Verification items for the finished model (mm, model axes). Face numbers are marked on the shaded views. Coordinates: 2 decimals unless noted, no trailing zeros. Loops run counter-clockwise (first coordinate to the right, second up) from the corner with the lowest first, then second, coordinate; pieces in that order, holes last. Notation, with made-up numbers: (37.25, 65) - (52.25, 65) arc R19 cw to (52.25, 69) - close; hole circle Ø7 at (-25, -8). An arc over 180 degrees is marked (long way). Answer as CSV lines item,"result". Start each with the question number.
1. Release check for a two-part mould opening along Y. For the marked faces 1 and 2 record: pulls with the +Y half, pulls with the -Y half, needs draft (parallel to the pull), parting line crosses it, or undercut.
2. Cross-section at B-B (z = -2). Enter the section's corners in (x, y).
3. Cross-section at A-A (y = 1460). State how many separate pieces and enclosed holes the cut face has, plus the area to 3 significant figures.
4. Material ranges on line 1 (Y direction, x = -53, z = -130); line 2 (Y direction, x = 55.5, z = 9.5); line 3 (Z direction, x = 56.5, y = 1460), recorded low to high. Write a range as [from, to].
5. Cross-section at C-C (x = 10). Enter the section's corners in (y, z), plus the area to 3 significant figures.
6. Gauge pin test, flat ends, axial feed: P1, Ø5, axis at x = 56, z = 14, coming from the -Y side; P2, Ø8, axis at y = 513, z = -42.5, coming from the +X side; P3, Ø4, axis at x = -22.5, y = 675.5, coming from the -Z side; P4, Ø11, axis at x = -52.5, z = -0.5, coming from the +Y side. Record the tip position at first contact, or that the pin passes through.
7. Cross-section at D-D (y = 587.5). Enter the section's corners in (x, z).
```python
from build123d import *

# Parameters (mm, degrees)
BOSS_EXTRUDE1_DEPTH = 2060
SKETCH2_R           = 17.5
BOSS_EXTRUDE2_DEPTH = 10
SKETCH4_R           = 17.5
BOSS_EXTRUDE3_DEPTH = 10


with BuildPart() as part:
    # Sketch1 → Boss-Extrude1 (new body)
    with BuildSketch(Plane(origin=(0, 0, 0), x_dir=(1, 0, 0), z_dir=(0, 1, 0))):
        with BuildLine():
            Line((-45, -75), (45, -75))
            ThreePointArc((45, -75), (48.535533906, -73.535533906), (50, -70))
            Line((50, -70), (50, 70))
            ThreePointArc((50, 70), (48.535533906, 73.535533906), (45, 75))
            Line((45, 75), (-45, 75))
            ThreePointArc((-45, 75), (-48.535533906, 73.535533906), (-50, 70))
            Line((-50, 70), (-50, -70))
            ThreePointArc((-50, -70), (-48.535533906, -73.535533906), (-45, -75))
        make_face()
        with BuildLine():
            Line((-30, -60), (30, -60))
            ThreePointArc((30, -60), (33.535533906, -58.535533906), (35, -55))
            Line((35, -55), (35, 55))
            ThreePointArc((35, 55), (33.535533906, 58.535533906), (30, 60))
            Line((30, 60), (-30, 60))
            ThreePointArc((-30, 60), (-33.535533906, 58.535533906), (-35, 55))
            Line((-35, 55), (-35, -55))
            ThreePointArc((-35, -55), (-33.535533906, -58.535533906), (-30, -60))
        make_face(mode=Mode.SUBTRACT)
    extrude(amount=BOSS_EXTRUDE1_DEPTH)

    # Sketch2 → Boss-Extrude2 (add)
    with BuildSketch(Plane(origin=(50, 0, 0), x_dir=(0, 0, -1), z_dir=(1, 0, 0))):
        with BuildLine():
            Line((43.395359238, 1396.045447211), (139.154011501, 1415.94090249))
            ThreePointArc((139.154011501, 1415.94090249), (175, 1460), (139.154011501, 1504.05909751))
            Line((139.154011501, 1504.05909751), (43.395359238, 1523.954552789))
            ThreePointArc((43.395359238, 1523.954552789), (38.336590995, 1524.737951503), (33.224235348, 1525))
            Line((33.224235348, 1525), (-56.636474138, 1525))
            Line((-56.636474138, 1525), (-56.636474138, 1460))
            Line((-56.636474138, 1460), (-56.636474138, 1395))
            Line((-56.636474138, 1395), (33.224235348, 1395))
            ThreePointArc((33.224235348, 1395), (38.336590995, 1395.262048497), (43.395359238, 1396.045447211))
        make_face()
        with Locations((130, 1460)):
            Circle(SKETCH2_R, mode=Mode.SUBTRACT)
        with BuildLine():
            Line((-56.636474138, 200), (-56.636474138, 265))
            Line((-56.636474138, 265), (104.432577767, 265))
            ThreePointArc((104.432577767, 265), (110.295724617, 264.655045152), (116.07797063, 263.624940361))
            Line((116.07797063, 263.624940361), (219.31631429, 238.899952288))
            ThreePointArc((219.31631429, 238.899952288), (250, 200), (219.31631429, 161.100047712))
            Line((219.31631429, 161.100047712), (116.07797063, 136.375059639))
            ThreePointArc((116.07797063, 136.375059639), (110.295724617, 135.344954848), (104.432577767, 135))
            Line((104.432577767, 135), (-56.636474138, 135))
            Line((-56.636474138, 135), (-56.636474138, 200))
        make_face()
        with Locations((210, 200)):
            Circle(SKETCH2_R, mode=Mode.SUBTRACT)
    extrude(amount=BOSS_EXTRUDE2_DEPTH)

    # Sketch4 → Boss-Extrude3 (add)
    with BuildSketch(Plane.ZY.offset(50)):
        with BuildLine():
            Line((-219.31631429, 238.899952288), (-109.901430019, 263.757549946))
            ThreePointArc((-109.901430019, 263.757549946), (-104.397629265, 264.688416645), (-98.824367082, 265))
            Line((-98.824367082, 265), (56.64, 265))
            Line((56.64, 265), (56.64, 200))
            Line((56.64, 200), (56.64, 135))
            Line((56.64, 135), (-98.824367082, 135))
            ThreePointArc((-98.824367082, 135), (-104.397629265, 135.311583355), (-109.901430019, 136.242450054))
            Line((-109.901430019, 136.242450054), (-219.31631429, 161.100047712))
            ThreePointArc((-219.31631429, 161.100047712), (-250, 200), (-219.31631429, 238.899952288))
        make_face()
        with Locations((-210, 200)):
            Circle(SKETCH4_R, mode=Mode.SUBTRACT)
        with BuildLine():
            Line((56.64, 1460), (56.64, 1525))
            Line((56.64, 1525), (-33.220885504, 1525))
            ThreePointArc((-33.220885504, 1525), (-38.333067886, 1524.737969312), (-43.391668321, 1523.954623652))
            Line((-43.391668321, 1523.954623652), (-139.154011501, 1504.05909751))
            ThreePointArc((-139.154011501, 1504.05909751), (-175, 1460), (-139.154011501, 1415.94090249))
            Line((-139.154011501, 1415.94090249), (-43.391668321, 1396.045376348))
            ThreePointArc((-43.391668321, 1396.045376348), (-38.333067886, 1395.262030688), (-33.220885504, 1395))
            Line((-33.220885504, 1395), (56.64, 1395))
            Line((56.64, 1395), (56.64, 1460))
        make_face()
        with Locations((-130, 1460)):
            Circle(SKETCH4_R, mode=Mode.SUBTRACT)
    extrude(amount=BOSS_EXTRUDE3_DEPTH)


solid = part.part
```
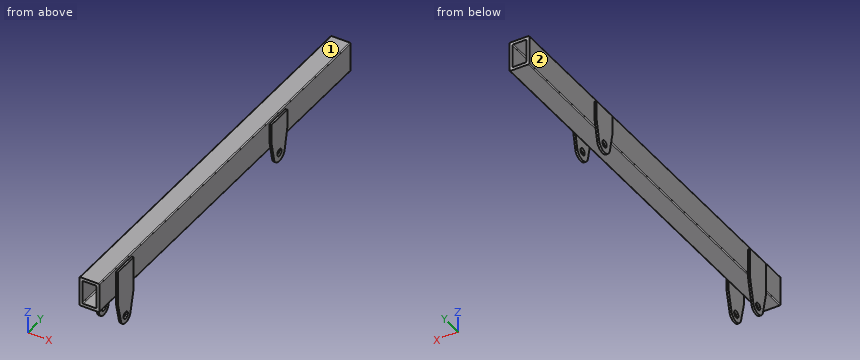
Values follow:
1,face 1,"needs draft"
1,face 2,"undercut"
2,outline,"(-60, 135) - (-50, 135) - (-50, 0) - (-35, 0) - (-35, 2060) - (-50, 2060) - (-50, 1525) - (-60, 1525) - (-60, 1395) - (-50, 1395) - (-50, 265) - (-60, 265) - close; (35, 0) - (50, 0) - (50, 135) - (60, 135) - (60, 265) - (50, 265) - (50, 1395) - (60, 1395) - (60, 1525) - (50, 1525) - (50, 2060) - (35, 2060) - close"
3,separate pieces,"3"
3,enclosed holes,"1"
3,area,"10,500 mm²"
4,line 1,"y = [140.81, 259.19], [1414.04, 1442.5], [1477.5, 1505.96]"
4,line 2,"y = [135, 265], [1395, 1525]"
4,line 3,"z = [-175, -147.5], [-112.5, 56.64]"
5,outline,"(0, -75) - (2060, -75) - (2060, -60) - (0, -60) - close; (0, 60) - (2060, 60) - (2060, 75) - (0, 75) - close"
5,area,"61,800 mm²"
6,P1,"stops at y = 135"
6,P2,"stops at x = 50"
6,P3,"stops at z = -75"
6,P4,"stops at y = 2060"
7,outline,"(-50, -70) arc R5 ccw to (-45, -75) - (45, -75) arc R5 ccw to (50, -70) - (50, 70) arc R5 ccw to (45, 75) - (-45, 75) arc R5 ccw to (-50, 70) - close; hole (-35, -55) arc R5 ccw to (-30, -60) - (30, -60) arc R5 ccw to (35, -55) - (35, 55) arc R5 ccw to (30, 60) - (-30, 60) arc R5 ccw to (-35, 55) - close"
